Autodesk Inventor part; units mm, degrees
ref_plane "YZ Plane" through (0, 0, 0) normal (1, 0, 0) x (0, 1, 0)
ref_plane "XZ Plane" through (0, 0, 0) normal (0, 1, 0) x (-1, 0, 0)
ref_plane "XY Plane" through (0, 0, 0) normal (0, 0, 1) x (1, 0, 0)
sketch "Boceto1" plane through (0, 0, 0) normal (0, 1, 0) x (-1, 0, 0)
  circle A0 centre (0, 0) radius 5
  circle A1 centre (-12.5, 0) radius 2.3
  dimension "d0" = 10
  dimension "d1" = 4.6
extrude "Extrusión1" add sketch "Boceto1" along normal blind 10.8
sketch "Boceto2" plane through (0, 10.8, 0) normal (0, 1, 0) x (1, 0, 0)
  circle A0 centre (0, 0) radius 5
  line L0 (30, 0) -> (30, -10)
  line L1 (-0.4927, -4.9757) -> (30, -7.9951)
  line L2 (30, 0) -> (30, 10)
  line L3 (-0.4927, 4.9757) -> (30, 7.9951)
extrude "Extrusión2" add sketch "Boceto2" along normal blind 10
sketch "Boceto3" plane through (0, 0, 0) normal (0, -1, 0) x (1, 0, 0)
  line L0 (30, -7.9951) -> (-0.4927, -4.9757)
  line L1 (30, 7.9951) -> (30, -7.9951)
  line L2 (-0.4927, 4.9757) -> (30, 7.9951)
  circle A0 centre (0, 0) radius 5
extrude "Extrusión3" add sketch "Boceto3" along normal blind 10
sketch "Boceto4" plane through (30, 10.8, 7.9951) normal (1, 0, 0) x (0, 0, -1)
  line L0 (0, 0) -> (15.9902, 0)
  line L1 (7.9951, 0) -> (7.9951, -10.8) construction
  line L2 (32.9951, 19.6) -> (-17.0049, 19.6)
  line L3 (-17.0049, 19.6) -> (-17.0049, -30.4)
  line L4 (-17.0049, -30.4) -> (32.9951, -30.4)
  line L5 (32.9951, -30.4) -> (32.9951, 19.6)
  line L6 (32.9951, 19.6) -> (-17.0049, -30.4) construction
  line L7 (-17.0049, 19.6) -> (32.9951, -30.4) construction
  point P0 (7.9951, -5.4)
  dimension "d10" = 50
  dimension "d11" = 50
extrude "Extrusión4" add sketch "Boceto4" along normal blind 10
properties part number "Pieza2PrimerEslabon" material "Cristal"
Can you work these out from the model? Positions are in its coordinate system, mm. A direction names the side the tool comes from. Coordinates: 2 decimals unless noted, no trailing zeros. Order: outer loops, then holes, each group sorted by start corner. A loop starts at its lowest first (then second) coordinate and runs counter-clockwise, first axis right, second up. Notation, with made-up numbers: M 16.5,-17 L 53.5,-17 A31 ccw 53.5,10 Z; hole C 55,72.5 d5. An arc over 180 degrees is marked long. Answer as CSV lines item,"result".
(1) Suppose I cut it at D-D on z = -13. Please give me the cut outline in (x, y).
Geometry check:
outline,"M 30,-19.6 L 40,-19.6 L 40,30.4 L 30,30.4 Z"
(2) Suppose I cut it at C-C on y = -12.5. Please give me the cut outline in (x, z).
Geometry check:
outline,"M 30,-25 L 40,-25 L 40,25 L 30,25 Z"
(3) Please list where these lines run through material, in increasing order: L1, parallel to Y at x = 21, z = -7; L2, parallel to X at y = 7.5, z = 21; L3, parallel to Y at x = 2, z = 3.
Geometry check:
L1,"-10 to 0, 10.8 to 20.8"
L2,"30 to 40"
L3,"-10 to 20.8"
(4) Suppose I cut it at B-B on x = 15.5. Please give me the cut outline in (y, z).
Geometry check:
outline,"M -10,-6.56 L 0,-6.56 L 0,6.56 L -10,6.56 Z; M 10.8,-6.56 L 20.8,-6.56 L 20.8,6.56 L 10.8,6.56 Z"
(5) If we mould it in two halves opening along X, with no side actions, what happens to faces 1 (the flat face through (18, 0, 0)), 2 (the flat face through (40, 6, 0)), 3 (the flat face through (35, 30.4, 0)), 4 (the flat face through (14.54, -4.93, 6.464))? For each: released by +X, released by -X, zero draft, split by the parting line, or undercut.
Geometry check:
face 1,"undercut"
face 2,"released by +X"
face 3,"zero draft"
face 4,"released by -X"
(6) I'm going to push flat-ended pins straight in: pin 1 (3 mm diameter, centred on x = 22.5, y = 14.5, fed in from +Z); pin 2 (8 mm diameter, centred on x = 14.5, z = -2, fed in from -Y); pin 3 (25 mm diameter, centred on y = -5.5, z = 2.5, fed in from -X); pin 4 (3 mm diameter, centred on x = 22.5, y = 20.5, fed in from -Z). Where does each tip first touch, or does it pass through?
Geometry check:
pin 1,"z = 7.4"
pin 2,"y = -10"
pin 3,"x = -5"
pin 4,"z = -7.4"
(7) Suppose I cut it at A-A on y = 1.5. Please give me the cut outline in (x, z), plus the area to 3 significant figures.
Geometry check:
outline,"C 0,0 d10; C 12.5,0 d4.6; M 30,-25 L 40,-25 L 40,25 L 30,25 Z"
area,"595 mm^2"
(8) On a 3-axis mill with a long thin cutter (end or side, diameter ignored), from which of +Z, -Z, +X, -X, +Y, -Y can I reach the whole of each face in a straight line? I mean faces 5 (the flat face through (12, 20.8, 0)), 6 (the cylindrical face through (14.798, 5.324, -0.101)), 7 (the flat face through (12, -10, 0)). Say none if no direction works.
Geometry check:
face 5,"+Z, -Z, -X, +Y"
face 6,"none"
face 7,"+Z, -Z, -X, -Y"
